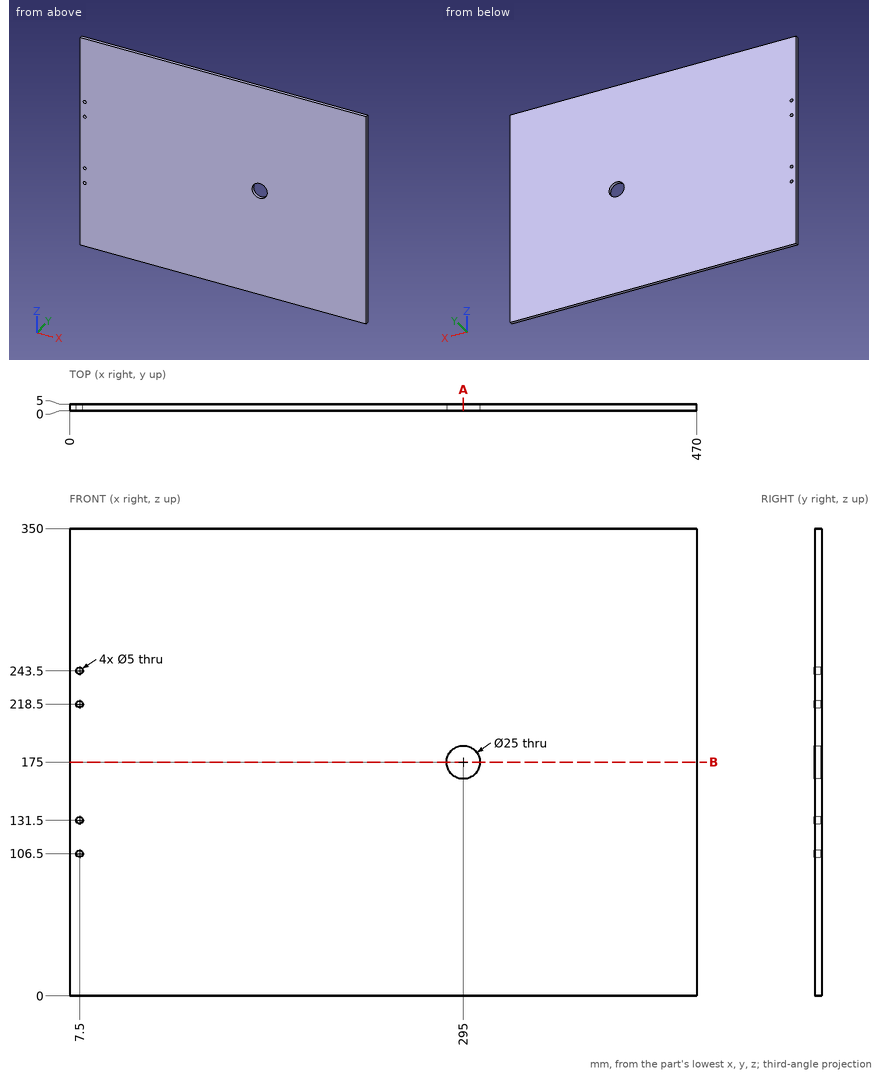
The figure shows three views and two pictorial views of one solid part (mm, origin at its lowest corner). Answer the questions. Give positions to 0.01 mm unless a question says otherwise; leave off trailing zeros. Order: outer loops, then holes, each group sorted by start corner. A loop starts at its lowest first (then second) coordinate and runs counter-clockwise, first axis right, second up. Notation, with made-up numbers: M 42.25,-27 L 82.25,-27 A18 cw 82.25,-9 Z; hole C 15.25,56 d8. An arc over 180 degrees is marked long. Return JSON: item names as keys, results as strings.
Q1. Find the intervals of material crossed by line 1 along Z through (x, y) = (7.5, 2.15); line 2 along X through (y, z) = (3.6, 243.5); line 3 along X through (y, z) = (0.2, 170), in increasing order. Write a range as [from, to].
Answer below:
{"line 1": "z = [0, 104], [109, 129], [134, 216], [221, 241], [246, 350]", "line 2": "x = [0, 5], [10, 470]", "line 3": "x = [0, 283.54], [306.46, 470]"}
Q2. Find section B-B, the plane z = 175. Write down the section's boundary in (x, y).
Answer below:
{"outline": "M 0,0 L 282.5,0 L 282.5,5 L 0,5 Z; M 307.5,0 L 470,0 L 470,5 L 307.5,5 Z"}
Q3. Find section A-A, the plane x = 295. Write down the section's boundary in (y, z).
Answer below:
{"outline": "M 0,0 L 5,0 L 5,162.5 L 0,162.5 Z; M 0,187.5 L 5,187.5 L 5,350 L 0,350 Z"}
